Geometry check sheet. Reference: the model listing, model coordinates, mm. Face numbers are marked on the shaded views. A direction names the side the tool comes from. Coordinates: 2 decimals unless noted, no trailing zeros. Order: outer loops, then holes, each group sorted by start corner. A loop starts at its lowest first (then second) coordinate and runs counter-clockwise, first axis right, second up. Notation, with made-up numbers: (72.5, 4) - (104.5, 4) arc R22 ccw to (104.5, 32) - close; hole circle Ø1 at (12, -7). An arc over 180 degrees is marked (long way). Use CSV: the item, a comma, the result in double quotes. Start each with the question number.
1) Sectioned sample at D-D, the plane y = -0.25. Record the cut outline in (x, z), and give its area (3 significant figures).
2) Sectioned sample at A-A, the plane x = -5.5. Record the cut outline in (y, z), and give its area (3 significant figures).
3) Sectioned sample at C-C, the plane x = -2.5. Record the cut outline in (y, z).
4) Thickness scan on probe 1 along Y at (x, z) = (-2.5, 10); probe 2 along X at (y, z) = (4, 7.5); probe 3 along X at (y, z) = (1.5, 12). Record the ranges inside material, lowest first. Write a range as [from, to].
5) Sectioned sample at B-B, the plane z = 7.5. Record the cut outline in (x, y).
6) Depth check by flat-ended pin: P1, Ø2.5, axis at x = -5, z = 9.5, coming from the +Y side; P2, Ø1, axis at x = 4, y = -1, coming from the -Z side; P3, Ø2.5, axis at x = -3, z = 9, coming from the -Y side. Enter the tip coordinate at first touch or a pass-through.
7) Tool access check on the marked faces 1, 2 and 3. Record the directions out of +Z, -Z, +X, -X, +Y, -Y that give a thin tool (end or side, any length) a straight path to the whole face; none if there is none.
8) Draft check along X on the marked faces 4, 5, 6 and 7. Enter one of: released by +X, released by -X, zero draft, split by the parting line, or undercut.
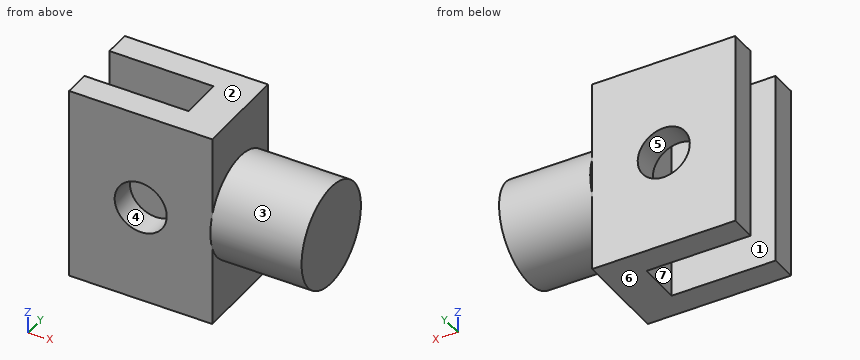
from build123d import *

# Parameters (mm, degrees)
BOSS_EXTRUDE1_DEPTH = 15
SKETCH5_R           = 2
CUT_EXTRUDE1_DEPTH  = 19.501081049
SKETCH4_R           = 3.9
BOSS_EXTRUDE2_DEPTH = 7


with BuildPart() as part:
    # Sketch1 → Boss-Extrude1 (new body)
    with BuildSketch(Plane.XY):
        Polygon((-8, 3.3), (-8, 5.3), (3, 5.3), (3, -2), (-8, -2), (-8, 0), (0, 0), (0, 3.3), align=None)
    extrude(amount=BOSS_EXTRUDE1_DEPTH)

    # Sketch5 → Cut-Extrude1 (cut, through all)
    with BuildSketch(Plane(origin=(0, 5.3, 0), x_dir=(1, 0, 0), z_dir=(0, 1, 0))):
        with Locations(Location((-2.5, -7.5, 0), (0, 0, 270))):
            Circle(SKETCH5_R)
    extrude(amount=-CUT_EXTRUDE1_DEPTH, mode=Mode.SUBTRACT)

    # Sketch4 → Boss-Extrude2 (add)
    with BuildSketch(Plane(origin=(3, 0, 0), x_dir=(0, 0, -1), z_dir=(1, 0, 0))):
        with Locations(Location((-7.5, 1.65, 0), (0, 0, 249.37361895))):
            Circle(SKETCH4_R)
    extrude(amount=BOSS_EXTRUDE2_DEPTH)


solid = part.part
Evaluation:
1,outline,"(-8, 0) - (3, 0) - (3, 4.09) - (10, 4.09) - (10, 10.91) - (3, 10.91) - (3, 15) - (-8, 15) - close; hole circle Ø4 at (-2.5, 7.5)"
1,area,"200 mm²"
2,outline,"(-2, 0) - (0, 0) - (0, 15) - (-2, 15) - close; (3.3, 0) - (5.3, 0) - (5.3, 15) - (3.3, 15) - close"
2,area,"60.0 mm²"
3,outline,"(-2, 0) - (0, 0) - (0, 5.5) - (-2, 5.5) - close; (-2, 9.5) - (0, 9.5) - (0, 15) - (-2, 15) - close; (3.3, 0) - (5.3, 0) - (5.3, 5.5) - (3.3, 5.5) - close; (3.3, 9.5) - (5.3, 9.5) - (5.3, 15) - (3.3, 15) - close"
4,probe 1,"[-2, 0], [3.3, 5.3]"
4,probe 2,"[-8, -4.5], [-0.5, 10]"
4,probe 3,"[0, 3]"
5,outline,"(-8, -2) - (-4.5, -2) - (-4.5, 0) - (-8, 0) - close; (-8, 3.3) - (-4.5, 3.3) - (-4.5, 5.3) - (-8, 5.3) - close; (-0.5, -2) - (3, -2) - (3, -2.25) - (10, -2.25) - (10, 5.55) - (3, 5.55) - (3, 5.3) - (-0.5, 5.3) - (-0.5, 3.3) - (0, 3.3) - (0, 0) - (-0.5, 0) - close"
6,P1,"y = 5.3"
6,P2,"z = 4.25"
6,P3,"y = -2"
7,face 1,"+Z, -Z, -X"
7,face 2,"+Z, +X, -X, +Y, -Y"
7,face 3,"+X"
8,face 4,"undercut"
8,face 5,"undercut"
8,face 6,"zero draft"
8,face 7,"released by -X"
